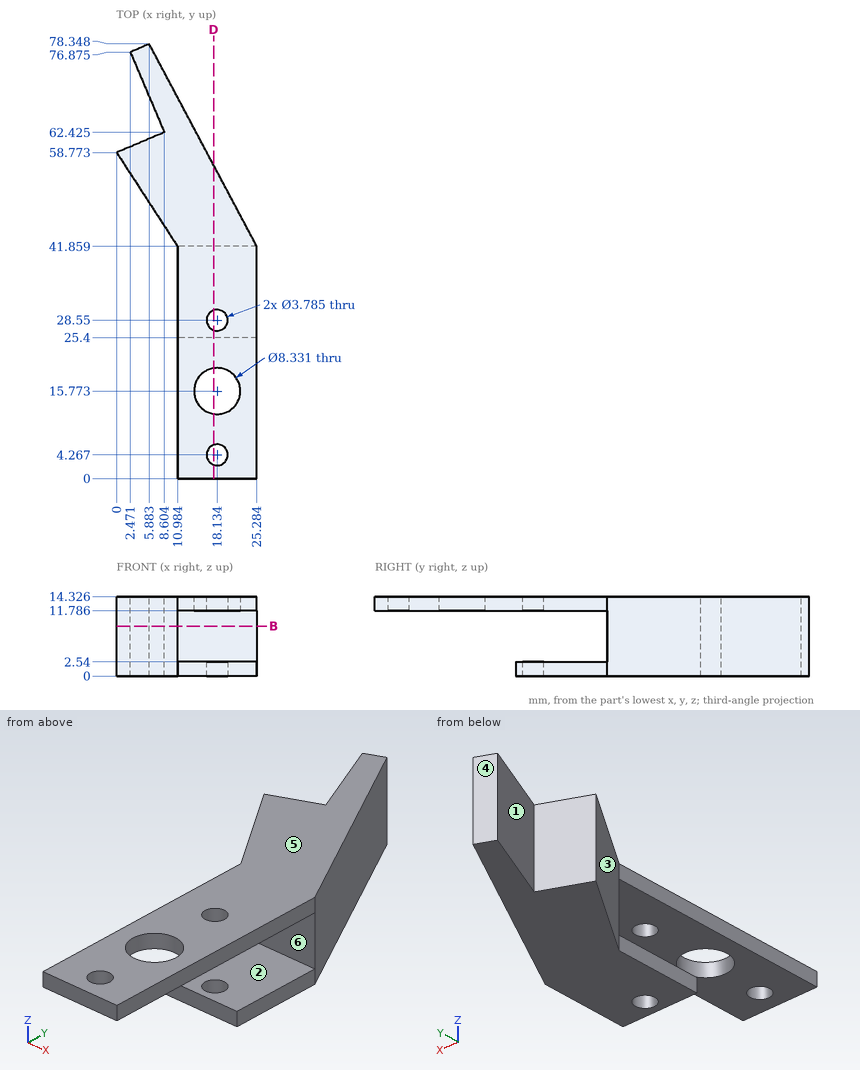
Geometry check sheet. Reference: drawing and pictorial views, mm from the part's lowest x, y, z. A direction names the side the tool comes from. Coordinates: 2 decimals unless noted, no trailing zeros. Write each loop counter-clockwise with the first axis right and the second up, starting at its lowest first coordinate (ties: lowest second). Pieces come first, ordered by that corner, then holes. Notation, with made-up numbers: M 43,9 L 67,9 A18 ccw 67,42 Z; hole C 26.5,-4.5 d5. An arc over 180 degrees is marked long. Write item = value, one per line. Start each with the question number.
1. Mould release check, pull along Z, two halves, no side actions. Record for the marked faces 4, 5 and 6: pulls with the +Z half, pulls with the -Z half, needs draft (parallel to the pull), parting line crosses it, or undercut.
2. Sectioned sample at B-B (z = 9). Record the cut outline in (x, y) (1 decimal), then the cut area to 3 significant figures.
3. Sectioned sample at D-D (x = 17.5). State how many separate pieces and enclosed holes the cut face has, then the cut area to 3 significant figures.
4. Tool access check on the marked faces 1, 2 and 3. Record the directions out of +Z, -Z, +X, -X, +Y, -Y that give a thin tool (end or side, any length) a straight path to the whole face; none if there is none.
5. Go/stop test with flat-tipped pins: pin 1 (3 mm diameter, centred on y = 21, z = 13.5, fed in from -X); pin 2 (1.3 mm diameter, centred on x = 18, z = 1, fed in from -Y); pin 3 (2 mm diameter, centred on x = 21, z = 4, fed in from -Y). Record where each tip stops, or that it passes through.
6. Thickness scan on probe 1 along Z at (x, y) = (15.5, 27.5) (1 decimal); probe 2 along X at (y, z) = (32.5, 2.25) (1 decimal); probe 3 along Y at (x, z) = (18, 2.25) (1 decimal). Record the ranges inside material, lowest first.
The answers:
q1.face_4 = needs draft
q1.face_5 = pulls with the +Z half
q1.face_6 = undercut
q2.outline = M 0,58.8 L 11,41.9 L 25.3,41.9 L 5.9,78.3 L 2.5,76.9 L 8.6,62.4 Z
q2.area = 374 mm²
q3.separate_pieces = 5
q3.enclosed_holes = 0
q3.area = 310 mm²
q4.face_1 = +Z, -Z, -X
q4.face_2 = +X, -X, -Y
q4.face_3 = +Z, -Z, -X, -Y
q5.pin_1 = 10.98
q5.pin_2 = 25.4
q5.pin_3 = 41.86
q6.probe_1 = 0 to 2.5, 11.8 to 14.3
q6.probe_2 = 11 to 25.3
q6.probe_3 = 25.4 to 26.7, 30.4 to 55.6
